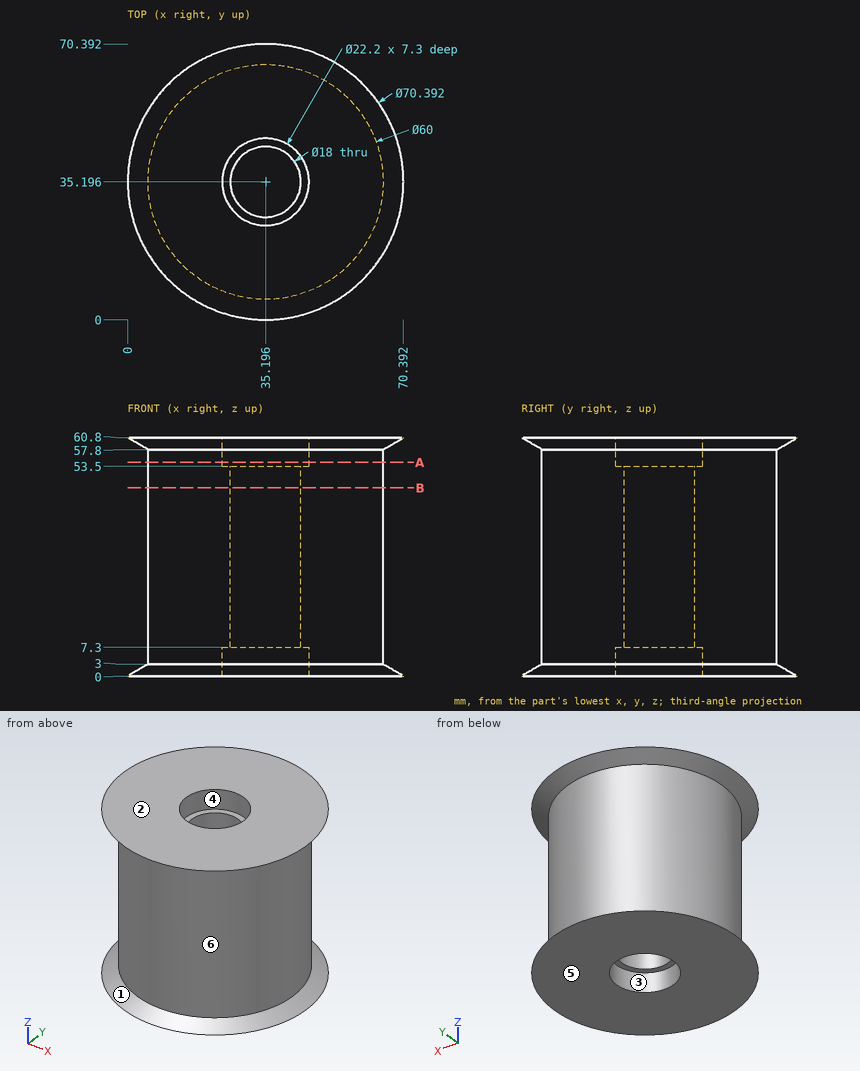
For this review, use the dimensioned drawing (mm, ordinates from the lowest corner) and the shaded views. A direction names the side the tool comes from. Round coordinates to 2 decimals unless told otherwise and drop trailing zeros. Order: outer loops, then holes, each group sorted by start corner. A loop starts at its lowest first (then second) coordinate and runs counter-clockwise, first axis right, second up. Notation, with made-up numbers: (42.5, -24.5) -> (57.5, -24.5) arc R14 ccw to (57.5, -14.5) -> close; hole circle Ø5 at (82, -38). An arc over 180 degrees is marked (long way). Put each result on its own line as item: value.
Q1. Mouldability with a two-part tool opening along Y and no side actions: class the marked faces 1, 2 and 3 as pulls with the +Y half, pulls with the -Y half, needs draft (parallel to the pull), parting line crosses it, or undercut.
Check result:
face 1: parting line crosses it
face 2: needs draft
face 3: undercut
Q2. Insertion check: pin 1 Ø3 at (y, z) = (53, 24) entering from +X; pin 2 Ø11 at (x, y) = (34, 30) entering from -Z; pin 3 Ø4 at (x, z) = (46, 29) entering from -Y. Each pin has a flat end and moves straight along its axis. Give the tip position at first contact, or say it passes through.
Check result:
pin 1: x = 60.38
pin 2: z = 7.3
pin 3: y = 6.52
Q3. Machinability: for the marked faces 4, 5 and 6, which of the approach directions +Z, -Z, +X, -X, +Y, -Y give a long, thin tool a straight path to every point of the face, cutting with its end or side? Answer none if there is none.
Check result:
face 4: +Z
face 5: -Z, +X, -X, +Y, -Y
face 6: none
Q4. Add section B-B on z = 48. Write out the cut boundary in (x, y).
Check result:
outline: circle Ø60 at (35.2, 35.2); hole circle Ø18 at (35.2, 35.2)
Q5. Add section A-A on z = 54.5. Write out the cut boundary in (x, y).
Check result:
outline: circle Ø60 at (35.2, 35.2); hole circle Ø22.2 at (35.2, 35.2)
Q6. For probe 1 along Y at (x, z) = (38.5, 45) (1 decimal); probe 2 along X at (y, z) = (34, 56); probe 3 along Z at (x, y) = (28.5, 41.5), list the stretches that pass through material, from the lowest coordinate up. Write a range as [from, to].
Check result:
probe 1: [5.4, 26.8], [43.6, 65]
probe 2: [5.22, 24.16], [46.23, 65.17]
probe 3: [7.3, 53.5]
